The listing builds one solid part. Answer for the finished solid, in the listing's coordinates (mm). Coordinates: 2 decimals unless noted, no trailing zeros. Write each loop counter-clockwise with the first axis right and the second up, starting at its lowest first coordinate (ties: lowest second). Pieces come first, ordered by that corner, then holes. Notation, with made-up numbers: M -2,52 L 7,52 A28 cw 7,82 Z; hole C 87.5,24.5 d10. An arc over 180 degrees is marked long. Answer as a JSON object with one key per item and string values. Group by question number.
from build123d import *

# Parameters (mm, degrees)
F1_DEPTH = 500


with BuildPart() as f1:
    # F0 (on Front) → F1 (new body, symmetric)
    with BuildSketch(Plane.XZ):
        with BuildLine():
            ThreePointArc((5, -6.2449979984), (7.2111025509, -3.4641016151), (8, 0))
            ThreePointArc((8, 0), (-3.4641016151, 7.2111025509), (-5, -6.2449979984))
            ThreePointArc((-5, -6.2449979984), (0, -8), (5, -6.2449979984))
        make_face()
        Polygon((5, -20), (-5, -20), (-20, -20), (-20, -25), (0, -25), (20, -25), (20, -20), align=None)
        with BuildLine():
            ThreePointArc((5, -6.2449979984), (0, -8), (-5, -6.2449979984))
            Line((-5, -6.2449979984), (-5, -20))
            Line((-5, -20), (5, -20))
            Line((5, -20), (5, -6.2449979984))
        make_face()
    extrude(amount=F1_DEPTH, both=True)


solid = f1.part
Item 1: A cutting plane is placed at B-B, the plane z = -11.5. Write down the section's boundary in (x, y), and give its area (3 significant figures).
Item 2: Consider L1, parallel to X at y = -135.5, z = -9; L2, parallel to Z at x = 14.5, y = -179.5; L3, parallel to Z at x = 0.5, y = 450. Determine where each line is inside the solid, lowest interval first. Write a range as from..to.
Item 3: A cutting plane is placed at A-A, the plane y = -220.5. Write down the section's boundary in (x, z) (3 decimals).
Item 4: A cutting plane is placed at C-C, the plane x = -14. Write down the section's boundary in (y, z), and give its area (3 significant figures).
Item 5: Flat-ended cylindrical pins translate along their axes: pin 1 Ø4 at (y, z) = (-154, -4.5) entering from +X; pin 2 Ø10 at (y, z) = (236.5, -7) entering from +X; pin 3 Ø2 at (y, z) = (12.5, -17.5) entering from -X. Find the tip coordinate at first contact, or state that the pin passes through.
Item 6: For a pull along Z with two mould halves and no side action, classify faces 1 (the face through (0, -7, 8)), 2 (the face through (0, -7, -25)), 3 (the face through (0, 500, -12)) as +Z half, -Z half, draft (parallel to the pull), parting line (faces both ways), or undercut.
Answer:
{
 "1": {"outline": "M -5,-500 L 5,-500 L 5,500 L -5,500 Z", "area": "10,000 mm2"},
 "2": {"L1": "-5..5", "L2": "-25..-20", "L3": "-25..7.98"},
 "3": {"outline": "M -20,-25 L 20,-25 L 20,-20 L 5,-20 L 5,-6.245 A8 ccw long -5,-6.245 L -5,-20 L -20,-20 Z"},
 "4": {"outline": "M -500,-25 L 500,-25 L 500,-20 L -500,-20 Z", "area": "5,000 mm2"},
 "5": {"pin 1": "x = 7.6", "pin 2": "x = 7.75", "pin 3": "x = -5"},
 "6": {"face 1": "undercut", "face 2": "-Z half", "face 3": "draft"}
}
